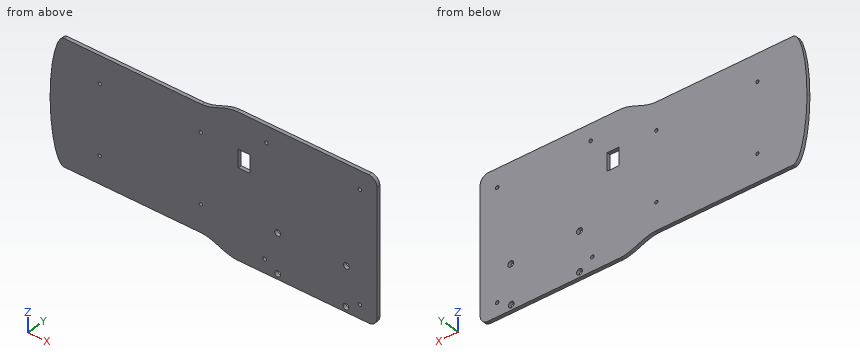
```python
from build123d import *

# Parameters (mm, degrees)
SKETCH_1_W           = 278
SKETCH_1_H           = 120
EXTRUDE_1_DEPTH      = 3
SKETCH_2_W           = 129
SKETCH_2_H           = 8
CUT_EXTRUDE_1_DEPTH  = 3
CUT_EXTRUDE_2_DEPTH  = 3
CUT_EXTRUDE_4_DEPTH  = 3
CUT_EXTRUDE_5_DEPTH  = 3
SKETCH_16_R          = 1.39979
CUT_EXTRUDE_9_DEPTH  = 10
SKETCH_18_W          = 10
SKETCH_18_H          = 15
CUT_EXTRUDE_10_DEPTH = 10
SKETCH_19_R          = 2.5
CUT_EXTRUDE_11_DEPTH = 10
SKETCH_20_R          = 1.5
CUT_EXTRUDE_12_DEPTH = 10
SKETCH_21_R          = 1.5
CUT_EXTRUDE_13_DEPTH = 10
SKETCH_22_R          = 2.5
CUT_EXTRUDE_14_DEPTH = 10
SKETCH_23_R          = 2.5
CUT_EXTRUDE_15_DEPTH = 10
SKETCH_24_R          = 1.5
CUT_EXTRUDE_16_DEPTH = 10
SKETCH_25_R          = 1.5
CUT_EXTRUDE_17_DEPTH = 10


with BuildPart() as part:
    # 스케치1 → 보스-돌출1 (new body)
    with BuildSketch(Plane(origin=(0, 0, 0), x_dir=(1, 0, 0), z_dir=(0, 1, 0))):
        Rectangle(SKETCH_1_W, SKETCH_1_H)
    extrude(amount=EXTRUDE_1_DEPTH)

    # 스케치2 → 컷-돌출1 (cut)
    with BuildSketch(Plane(origin=(0, 3, 0), x_dir=(1, 0, 0), z_dir=(0, 1, 0))):
        with Locations((-74.5, -56)):
            Rectangle(SKETCH_2_W, SKETCH_2_H)
        with Locations((-74.5, 56)):
            Rectangle(SKETCH_2_W, SKETCH_2_H)
    extrude(amount=-CUT_EXTRUDE_1_DEPTH, mode=Mode.SUBTRACT)

    # 스케치3 → 컷-돌출2 (cut)
    with BuildSketch(Plane(origin=(0, 3, 0), x_dir=(1, 0, 0), z_dir=(0, 1, 0))):
        with BuildLine():
            add(Edge.make_bspline(
                [(-127, 52), (-139, 52), (-139, 0)],
                knots=[3.141592654, 3.141592654, 3.141592654, 4.71238898, 4.71238898, 4.71238898], degree=2, weights=[1, 0.707106781, 1]))
            Line((-127, 52), (-139, 52))
            Line((-139, 52), (-139, 0))
        make_face()
        with BuildLine():
            Line((-139, -52), (-127, -52))
            add(Edge.make_bspline(
                [(-139, 0), (-139, -52), (-127, -52)],
                knots=[4.71238898, 4.71238898, 4.71238898, 6.283185307, 6.283185307, 6.283185307], degree=2, weights=[1, 0.707106781, 1]))
            Line((-139, 0), (-139, -52))
        make_face()
    extrude(amount=-CUT_EXTRUDE_2_DEPTH, mode=Mode.SUBTRACT)

    # 스케치4 → 컷-돌출4 (cut)
    with BuildSketch(Plane(origin=(0, 3, 0), x_dir=(1, 0, 0), z_dir=(0, 1, 0))):
        with BuildLine():
            Line((-10, 52), (-10, 60))
            Line((-10, 60), (20, 60))
            add(Edge.make_bspline(
                [(-10, 52), (0.64121866, 52.367223255), (9.376693721, 59.919927591), (20, 60)],
                knots=[0, 0, 0, 0, 1, 1, 1, 1], degree=3))
        make_face()
        with BuildLine():
            Line((-10, -52), (-10, -60))
            Line((-10, -60), (20, -60))
            add(Edge.make_bspline(
                [(-10, -52), (0.64121866, -52.367223255), (9.376693721, -59.919927591), (20, -60)],
                knots=[0, 0, 0, 0, 1, 1, 1, 1], degree=3))
        make_face()
    extrude(amount=-CUT_EXTRUDE_4_DEPTH, mode=Mode.SUBTRACT)

    # 스케치5 → 컷-돌출5 (cut)
    with BuildSketch(Plane(origin=(0, 3, 0), x_dir=(1, 0, 0), z_dir=(0, 1, 0))):
        with BuildLine():
            Line((132, 60), (139, 60))
            Line((139, 60), (139, 53))
            ThreePointArc((139, 53), (136.949747468, 57.949747468), (132, 60))
        make_face()
        with BuildLine():
            Line((139, -60), (139, -53))
            ThreePointArc((139, -53), (136.949747468, -57.949747468), (132, -60))
            Line((132, -60), (139, -60))
        make_face()
    extrude(amount=-CUT_EXTRUDE_5_DEPTH, mode=Mode.SUBTRACT)

    # 스케치16 → 컷-돌출9 (cut)
    with BuildSketch(Plane(origin=(0, 3, 0), x_dir=(1, 0, 0), z_dir=(0, 1, 0))):
        with Locations(Location((-96.85129, 29.0311, 0), (0, 0, 270))):
            Circle(SKETCH_16_R)
        with Locations(Location((-96.85109, -28.96802, 0), (0, 0, 270))):
            Circle(SKETCH_16_R)
        with Locations(Location((-10.85223, 29.03265, 0), (0, 0, 270))):
            Circle(SKETCH_16_R)
        with Locations(Location((-10.8511, -28.96784, 0), (0, 0, 270))):
            Circle(SKETCH_16_R)
    extrude(amount=-CUT_EXTRUDE_9_DEPTH, mode=Mode.SUBTRACT)

    # 스케치18 → 컷-돌출10 (cut)
    with BuildSketch(Plane(origin=(0, 3, 0), x_dir=(1, 0, 0), z_dir=(0, 1, 0))):
        with Locations((26, -22.5)):
            Rectangle(SKETCH_18_W, SKETCH_18_H)
    extrude(amount=-CUT_EXTRUDE_10_DEPTH, mode=Mode.SUBTRACT)

    # 스케치19 → 컷-돌출11 (cut)
    with BuildSketch(Plane(origin=(0, 3, 0), x_dir=(1, 0, 0), z_dir=(0, 1, 0))):
        with Locations(Location((112.6, 55.5, 0), (0, 0, 270))):
            Circle(SKETCH_19_R)
    extrude(amount=-CUT_EXTRUDE_11_DEPTH, mode=Mode.SUBTRACT)

    # 스케치20 → 컷-돌출12 (cut)
    with BuildSketch(Plane(origin=(0, 3, 0), x_dir=(1, 0, 0), z_dir=(0, 1, 0))):
        with Locations(Location((124.5, 48.5, 0), (0, 0, 270))):
            Circle(SKETCH_20_R)
    extrude(amount=-CUT_EXTRUDE_12_DEPTH, mode=Mode.SUBTRACT)

    # 스케치21 → 컷-돌출13 (cut)
    with BuildSketch(Plane(origin=(0, 3, 0), x_dir=(1, 0, 0), z_dir=(0, 1, 0))):
        with Locations(Location((124.5, -44.5, 0), (0, 0, 270))):
            Circle(SKETCH_21_R)
    extrude(amount=-CUT_EXTRUDE_13_DEPTH, mode=Mode.SUBTRACT)

    # 스케치22 → 컷-돌출14 (cut)
    with BuildSketch(Plane(origin=(0, 3, 0), x_dir=(1, 0, 0), z_dir=(0, 1, 0))):
        with Locations(Location((54.5, 55.5, 0), (0, 0, 270))):
            Circle(SKETCH_22_R)
    extrude(amount=-CUT_EXTRUDE_14_DEPTH, mode=Mode.SUBTRACT)

    # 스케치23 → 컷-돌출15 (cut)
    with BuildSketch(Plane(origin=(0, 3, 0), x_dir=(1, 0, 0), z_dir=(0, 1, 0))):
        with Locations(Location((113, 22.5, 0), (0, 0, 270))):
            Circle(SKETCH_23_R)
        with Locations(Location((54.5, 22.5, 0), (0, 0, 270))):
            Circle(SKETCH_23_R)
    extrude(amount=-CUT_EXTRUDE_15_DEPTH, mode=Mode.SUBTRACT)

    # 스케치24 → 컷-돌출16 (cut)
    with BuildSketch(Plane(origin=(0, 3, 0), x_dir=(1, 0, 0), z_dir=(0, 1, 0))):
        with Locations(Location((45, -46, 0), (0, 0, 270))):
            Circle(SKETCH_24_R)
    extrude(amount=-CUT_EXTRUDE_16_DEPTH, mode=Mode.SUBTRACT)

    # 스케치25 → 컷-돌출17 (cut)
    with BuildSketch(Plane(origin=(0, 3, 0), x_dir=(1, 0, 0), z_dir=(0, 1, 0))):
        with Locations(Location((43.5, 48.5, 0), (0, 0, 270))):
            Circle(SKETCH_25_R)
    extrude(amount=-CUT_EXTRUDE_17_DEPTH, mode=Mode.SUBTRACT)


solid = part.part
```
Verification items for the finished model (mm, model axes). Coordinates: 2 decimals unless noted, no trailing zeros. Loops run counter-clockwise (first coordinate to the right, second up) from the corner with the lowest first, then second, coordinate; pieces in that order, holes last. Notation, with made-up numbers: (10.5, -28.75) - (31.5, -28.75) arc R36 ccw to (31.5, 5.25) - close; hole circle Ø3 at (71, -1). An arc over 180 degrees is marked (long way). Put each result on its own line as item: value.
Item 1: Scan lines: line 1 along Z through (x, y) = (124.5, 1.15); line 2 along X through (y, z) = (1.7, -28); line 3 along X through (y, z) = (1.55, 45). Record each from-to range of solid material in increasing order.
Conclusion:
line 1: z = -60 to -50, -47 to 43, 46 to 60
line 2: x = -137.11 to -97.8, -95.9 to -11.8, -9.91 to 139
line 3: x = -133.01 to 43.88, 46.12 to 123.09, 125.91 to 139
Item 2: Gauge pin test, flat ends, axial feed: pin 1 Ø1.5 at (x, y) = (-66, 1.5) entering from -Z; pin 2 Ø3.5 at (x, z) = (45, 46) entering from -Y; pin 3 Ø1 at (y, z) = (1, 40) entering from -X; pin 4 Ø2.5 at (x, z) = (-10.85, -29.03) entering from +Y. Record the tip position at first contact, or that the pin passes through.
Conclusion:
pin 1: stops at z = -52
pin 2: stops at y = 0
pin 3: stops at x = -134.8
pin 4: passes through
Item 3: Section check A-A (x = -83.5). Enter the section's corners in (y, z).
Conclusion:
outline: (0, -52) - (3, -52) - (3, 52) - (0, 52) - close
Item 4: Section check B-B (y = 2.25). Give the number of separate pieces and of enclosed holes in the cut face, then the cut area to 3 significant figures.
Conclusion:
separate pieces: 1
enclosed holes: 13
area: 30,500 mm2
